Autodesk Inventor part; units mm, degrees
ref_plane "YZ Plane" through (0, 0, 0) normal (1, 0, 0) x (0, 1, 0)
ref_plane "XZ Plane" through (0, 0, 0) normal (0, 1, 0) x (-1, 0, 0)
ref_plane "XY Plane" through (0, 0, 0) normal (0, 0, 1) x (1, 0, 0)
sketch "Szkic1" plane through (0, 0, 0) normal (0, 0, 1) x (1, 0, 0)
  line L0 (2.3165, 0) -> (0.0582, 0) construction
  arc A0 (1.1874, -2.3597) -> (2.3165, 0) centre (1.1874, -0.9097) ccw construction
  arc A1 (0.0582, 0) -> (1.1874, -2.3597) centre (1.1874, -0.9097) ccw construction
  circle A2 centre (1.1874, -0.9097) radius 10.5
  line L1 (-0.0447, 0.225) -> (2.4195, 0.225)
  arc A3 (2.8624, -0.9097) -> (2.4195, 0.225) centre (1.1874, -0.9097) ccw
  arc A4 (-0.0447, 0.225) -> (2.8624, -0.9097) centre (1.1874, -0.9097) ccw
  circle A5 centre (1.1874, -0.9097) radius 8.5
  point P0 (0, 0)
  dimension "d0" = 21
  dimension "d7" = 1.45
  dimension "d8" = 0.225
  dimension "d9" = 17
extrude "Wyciągnięcie proste1" add sketch "Szkic1" along normal blind 7 contours A2 | A5
sketch "Szkic3" plane through (1.1874, -0.9097, 0) normal (0, 0, -1) x (-1, 0, 0)
  point P0 (1.1874, 0.9097)
extrude "Wyciągnięcie proste3" add sketch "Szkic1" against normal blind 5 contours A2
properties part number "felga"
For this review, take the finished solid that the model builds, in its own axes (mm). A direction names the side the tool comes from. Round coordinates to 2 decimals unless told otherwise and drop trailing zeros. Order: outer loops, then holes, each group sorted by start corner. A loop starts at its lowest first (then second) coordinate and runs counter-clockwise, first axis right, second up.
Q1. We need section C-C, the plane x = 1. Give the boundary of the cut face in (y, z) (3 decimals).
Findings below:
outline: (-11.408, -5) - (-9.408, -5) - (-9.408, 0) - (-2.574, 0) - (-2.574, 7) - (-11.408, 7) - close; (0.225, 0) - (7.588, 0) - (7.588, -5) - (9.589, -5) - (9.589, 7) - (0.225, 7) - close
Q2. Machinability: for faces 1 (the cylindrical face through (-0.655, -9.208, -2.465)), 2 (the flat face through (10, -1, -5)), 3 (the flat face through (1, 0.225, 3)), which of the approach directions +Z, -Z, +X, -X, +Y, -Y give a long, thin tool a straight path to every point of the face, cutting with its end or side? Answer none if there is none.
Findings below:
face 1: -Z
face 2: -Z, +X, -X, +Y, -Y
face 3: +Z, -Z
Q3. Insertion check: P1, Ø4, axis at y = -8.5, z = -1.5, coming from the +X side; P2, Ø6, axis at x = -7, z = 1.5, coming from the -Y side; P3, Ø1.5, axis at y = -7, z = 0, coming from the -X side. Each pin has a flat end and moves straight along its axis. Give the tip position at first contact, or say it passes through.
Findings below:
P1: stops at x = 10.08
P2: stops at y = -10.04
P3: stops at x = -7.85
Q4. We need section A-A, the plane y = -1.5. Give the boundary of the cut face in (x, z).
Findings below:
outline: (-9.3, -5) - (-7.29, -5) - (-7.29, 0) - (-0.38, 0) - (-0.38, 7) - (-9.3, 7) - close; (2.75, 0) - (9.67, 0) - (9.67, -5) - (11.67, -5) - (11.67, 7) - (2.75, 7) - close
Q5. We need section B-B, the plane x = -2.25. Give the boundary of the cut face in (y, z), plus the area to 3 significant figures.
Findings below:
outline: (-10.83, -5) - (-8.68, -5) - (-8.68, 0) - (6.86, 0) - (6.86, -5) - (9.01, -5) - (9.01, 7) - (-10.83, 7) - close
area: 160 mm2
Q6. We need section D-D, the plane z = -1.25. Give the boundary of the cut face in (x, y).
Findings below:
outline: circle Ø21 at (1.19, -0.91); hole circle Ø17 at (1.19, -0.91)
Q7. Wall thickness on line 1 (Y direction, x = 1.25, z = 4.5) (3 decimals); line 2 (Z direction, x = 0.75, y = 6.25); line 3 (Y direction, x = -0.75, z = -1.25): over which ranges is each line inside the solid? List them lowest first.
Findings below:
line 1: y = -11.41 to -2.584, 0.225 to 9.59
line 2: z = 0 to 7
line 3: y = -11.23 to -9.19, 7.37 to 9.41
Q8. Mouldability with a two-part tool opening along Y and no side actions: class faces 4 (the cylindrical face through (2.745, -0.293, 3.451)), 5 (the flat face through (1, -3, 7)), 6 (the cylindrical face through (6.033, -10.225, 1.084)) as pulls with the +Y half, pulls with the -Y half, needs draft (parallel to the pull), parting line crosses it, or undercut.
Findings below:
face 4: undercut
face 5: needs draft
face 6: parting line crosses it
